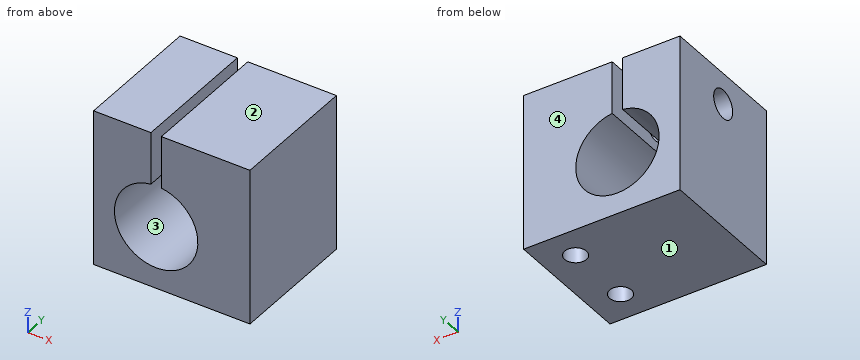
```python
from build123d import *

# Parameters (mm, degrees)
F1_DEPTH = 12.5
F3_D     = 5.5
F3_DEPTH = 12
F3_TIP   = 1.6523667023
F5_D     = 4.2
F5_DEPTH = 8
F5_TIP   = 1.2618073
F7_D     = 4.2
F7_DEPTH = 14
F7_TIP   = 1.2618073


with BuildPart() as f1:
    # F0 (on Front) → F1 (new body, symmetric)
    with BuildSketch(Plane.XZ):
        with BuildLine():
            Line((15, -15), (15, 15))
            Line((15, 15), (-2, 15))
            Line((-2, 15), (-2, 4.9372539332))
            ThreePointArc((-2, 4.9372539332), (-3, -11), (-4, 4.9372539332))
            Line((-4, 4.9372539332), (-4, 15))
            Line((-4, 15), (-15, 15))
            Line((-15, 15), (-15, -15))
            Line((-15, -15), (15, -15))
        make_face()
    extrude(amount=F1_DEPTH, both=True)

    # F3
    with Locations(Plane(origin=(-15, 0, 0), x_dir=(0, -1, 0), z_dir=(-1, 0, 0))):
        with Locations((0, 9)):
            Hole(F3_D / 2, depth=F3_DEPTH)
            with Locations((0, 0, -(F3_DEPTH + F3_TIP / 2))):  # 118° drill point
                Cone(0, F3_D / 2, F3_TIP, mode=Mode.SUBTRACT)

    # F5
    with Locations(Plane(origin=(-2, 0, 0), x_dir=(0, -1, 0), z_dir=(-1, 0, 0))):
        with Locations((0, 9)):
            Hole(F5_D / 2, depth=F5_DEPTH)
            with Locations((0, 0, -(F5_DEPTH + F5_TIP / 2))):  # 118° drill point
                Cone(0, F5_D / 2, F5_TIP, mode=Mode.SUBTRACT)

    # F7
    with Locations(Plane(origin=(0, 0, -15), x_dir=(1, 0, 0), z_dir=(0, 0, -1))):
        with Locations((9, 6.5), (9, -6.5)):
            Hole(F7_D / 2, depth=F7_DEPTH)
            with Locations((0, 0, -(F7_DEPTH + F7_TIP / 2))):  # 118° drill point
                Cone(0, F7_D / 2, F7_TIP, mode=Mode.SUBTRACT)


solid = f1.part
```
Source: CAD feature listing. Evaluate the final solid. Frame: model axes, mm. Face numbers are marked on the shaded views. Give positions to 0.01 mm unless a question says otherwise; leave off trailing zeros. Loops run counter-clockwise (first coordinate to the right, second up) from the corner with the lowest first, then second, coordinate; pieces in that order, holes last. Notation, with made-up numbers: (74, 11.25) - (113, 11.25) arc R33 ccw to (113, 50.25) - close; hole circle Ø10 at (-34.75, 60.25). An arc over 180 degrees is marked (long way). Use CSV: the item, a comma, the result in double quotes. Start each with the question number.
1. Pin query (flat end, axial travel): pin 1 (4 mm diameter, centred on x = 9, y = -6.5, fed in from -Z); pin 2 (1 mm diameter, centred on x = -3, z = 6.5, fed in from -Y); pin 3 (2.5 mm diameter, centred on y = 0, z = 9, fed in from -X). Return the tip coordinate at first contact, or that it passes through.
2. Section C-C (y = 3.25). Output: boundary loops of the cut face in (x, z), then the cut area to 3 significant figures.
3. Section A-A (z = -8.5). Output: boundary loops of the cut face in (x, y), then the cut area to 3 significant figures.
4. Section D-D (z = 3.5). Output: boundary loops of the cut face in (x, y), then the cut area to 3 significant figures.
5. Section B-B (x = 4.5). Output: boundary loops of the cut face in (y, z), then the cut area to 3 significant figures.
6. Ray query, L1, parallel to Y at x = 9, z = -11; L2, parallel to X at y = 4.5, z = 12.75; L3, parallel to Y at x = 0, z = 9. Return the intervals inside material, ascending.
7. Draft query along Z for the marked faces 1, 2, 3 and 4. Return one class per face: +Z half, -Z half, draft (parallel to the pull), parting line (faces both ways), or undercut.
Response:
1,pin 1,"z = -0.94"
1,pin 2,"through"
1,pin 3,"x = 6.51"
2,outline,"(-15, -15) - (15, -15) - (15, 15) - (-2, 15) - (-2, 4.94) arc R8 cw (long way) to (-4, 4.94) - (-4, 15) - (-15, 15) - close"
2,area,"679 mm²"
3,outline,"(-15, -12.5) - (-8.81, -12.5) - (-8.81, 12.5) - (-15, 12.5) - close; (2.81, -12.5) - (15, -12.5) - (15, 12.5) - (2.81, 12.5) - close; hole circle Ø4.2 at (9, -6.5); hole circle Ø4.2 at (9, 6.5)"
3,area,"432 mm²"
4,outline,"(-15, -12.5) - (-7.66, -12.5) - (-7.66, 12.5) - (-15, 12.5) - close; (1.66, -12.5) - (15, -12.5) - (15, 12.5) - (1.66, 12.5) - close"
4,area,"517 mm²"
5,outline,"(-12.5, -15) - (12.5, -15) - (12.5, -5.78) - (-12.5, -5.78) - close; (-12.5, -0.22) - (12.5, -0.22) - (12.5, 15) - (-12.5, 15) - close; hole circle Ø4.2 at (0, 9)"
5,area,"597 mm²"
6,L1,"-12.5 to -8.6, -4.4 to 4.4, 8.6 to 12.5"
6,L2,"-15 to -4, -2 to 15"
6,L3,"-12.5 to -2.1, 2.1 to 12.5"
7,face 1,"-Z half"
7,face 2,"+Z half"
7,face 3,"undercut"
7,face 4,"draft"
